Read the model definition and answer for the solid it produces. Units are mm, in the model's axes. Face numbers are marked on the shaded views. Round coordinates to 2 decimals unless told otherwise and drop trailing zeros. Order: outer loops, then holes, each group sorted by start corner. A loop starts at its lowest first (then second) coordinate and runs counter-clockwise, first axis right, second up. Notation, with made-up numbers: (9.25, 81.25) -> (53.25, 81.25) arc R27 ccw to (53.25, 105.25) -> close; hole circle Ø1 at (-12, -29.75). An arc over 180 degrees is marked (long way). Use a Markdown table: item, result. Add a question column.
1. Given pin 1 (2 mm diameter, centred on y = -1.5, z = -30, fed in from +X); pin 2 (7.5 mm diameter, centred on y = 1.5, z = -58, fed in from -X); pin 3 (4.5 mm diameter, centred on x = -55.5, y = 3, fed in from -Z), each flat-ended and moving along its own axis, determine where each tip first touches the part or whether it passes through.
2. Section A-A, the plane y = 0 is taken. Give the vertices of the cut face in (x, z), then the cut area to 3 significant figures.
3. The mould has two halves that part along X. Classify the marked faces 1, 2 and 3: +X half, -X half, draft (parallel to the pull), parting line (faces both ways), or undercut.
4. Section C-C, the plane y = 4.75 is taken. Give the vertices of the cut face in (x, z).
5. Section B-B, the plane x = -47 is taken. Give the vertices of the cut face in (y, z).
6. Section D-D, the plane z = -32 is taken. Give the vertices of the cut face in (x, y).
7. Consider L1, parallel to Z at x = -42.65, y = 0; L2, parallel to X at y = 5.25, z = -54; L3, parallel to Z at x = -61.15, y = 0. Determine where each line is inside the solid, lowest interval first. Write a range as [from, to].
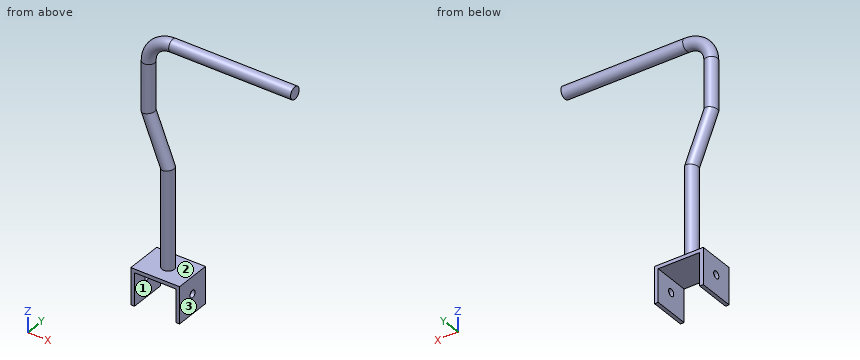
```python
from build123d import *

# Parameters (mm, degrees)
F1_R     = 2.5
F4_W     = 15
F4_H     = 15
F5_DEPTH = 10
F6_W     = 17
F6_H     = 13.5
F7_DEPTH = 25
F8_R     = 1.5
F9_DEPTH = 25


with BuildPart() as f2:
    # F2: sweep along a path in F0
    with BuildLine(Plane.XZ) as f2_path:
        Line((0, 39.5429997165), (-50, 39.5429997165))
        ThreePointArc((-50, 39.5429997165), (-57.0710678119, 36.6140675284), (-60, 29.5429997165))
        Line((-60, 29.5429997165), (-60, 9.5429997165))
        Line((-60, 9.5429997165), (-52, -10.4570002835))
        Line((-52, -10.4570002835), (-52, -50.4570002835))
    # F1 (on Right) → F2 (sweep)
    with BuildSketch(Plane.YZ):
        with Locations((0, 39.5429997165)):
            Circle(F1_R)
    sweep(path=f2_path.line, transition=Transition.RIGHT)

    # F4 (on offset) → F5 (join, symmetric)
    with BuildSketch(Plane.YZ.offset(-52)):
        with Locations((0, -57.9570002835)):
            Rectangle(F4_W, F4_H)
    extrude(amount=F5_DEPTH, both=True)

    # F6 (on face) → F7 (cut)
    with BuildSketch(Plane.XZ.offset(7.5)):
        with Locations((-52, -58.7070002835)):
            Rectangle(F6_W, F6_H)
    extrude(amount=-F7_DEPTH, mode=Mode.SUBTRACT)

    # F8 (on face) → F9 (cut)
    with BuildSketch(Plane(origin=(-62, 0, 0), x_dir=(0, -1, 0), z_dir=(-1, 0, 0))):
        with Locations((0, -57.4570002835)):
            Circle(F8_R)
    extrude(amount=-F9_DEPTH, mode=Mode.SUBTRACT)


solid = f2.part
```
Verdict:
| question | item | result |
|---|---|---|
| 1 | pin 1 | stops at x = -49.55 |
| 1 | pin 2 | stops at x = -62 |
| 1 | pin 3 | stops at z = -51.96 |
| 2 | outline | (-62.5, 9.06) -> (-54.5, -10.94) -> (-54.5, -50.46) -> (-62, -50.46) -> (-62, -55.96) -> (-60.5, -55.96) -> (-60.5, -51.96) -> (-43.5, -51.96) -> (-43.5, -55.96) -> (-42, -55.96) -> (-42, -50.46) -> (-49.5, -50.46) -> (-49.5, -9.98) -> (-57.5, 10.02) -> (-57.5, 29.54) arc R7.5 cw to (-50, 37.04) -> (0, 37.04) -> (0, 42.04) -> (-50, 42.04) arc R12.5 ccw to (-62.5, 29.54) -> close; (-62, -65.46) -> (-60.5, -65.46) -> (-60.5, -58.96) -> (-62, -58.96) -> close; (-43.5, -65.46) -> (-42, -65.46) -> (-42, -58.96) -> (-43.5, -58.96) -> close |
| 2 | area | 798 mm2 |
| 3 | face 1 | undercut |
| 3 | face 2 | draft |
| 3 | face 3 | +X half |
| 4 | outline | (-62, -65.46) -> (-60.5, -65.46) -> (-60.5, -51.96) -> (-43.5, -51.96) -> (-43.5, -65.46) -> (-42, -65.46) -> (-42, -50.46) -> (-62, -50.46) -> close |
| 5 | outline | (-7.5, -51.96) -> (7.5, -51.96) -> (7.5, -50.46) -> (-7.5, -50.46) -> close; circle Ø5 at (0, 39.54) |
| 6 | outline | circle Ø5 at (-52, 0) |
| 7 | L1 | z = [-65.46, -58.96], [-55.96, -50.46], [37.04, 42.04] |
| 7 | L2 | x = [-62, -60.5], [-43.5, -42] |
| 7 | L3 | z = [-65.46, -58.96], [-55.96, -50.46], [5.69, 35.19] |
